```python
from build123d import *

# Parameters (mm, degrees)
F0_W     = 129.536152
F0_H     = 24.80902
F2_DEPTH = 2
F1_W     = 2.46322
F1_H     = 3.985553
F1_W_2   = 9.229143
F1_H_2   = 15.286758
F1_W_3   = 2.812087
F1_H_3   = 9.482866
F1_W_4   = 2.463219
F1_H_4   = 5.571315
F3_DEPTH = 1.5


with BuildPart() as f2:
    # F0 (on Top) → F2 (new body)
    with BuildSketch(Plane.XY):
        Rectangle(F0_W, F0_H)
    extrude(amount=-F2_DEPTH)

    # F1 (on Top) → F3 (join)
    with BuildSketch(Plane.XY):
        Polygon((-53.720365, 7.334459), (-53.720365, -1.440098), (-56.82846, 7.334459), (-59.999987, 7.334459), (-59.999987, -7.952299), (-56.997608, -7.952299), (-56.997608, 0.822258), (-53.868369, -7.952299), (-50.696842, -7.952299), (-50.696842, 7.334459), align=None)
        Polygon((-43.87806, -7.952299), (-43.87806, -5.055639), (-44.935236, -5.055639), (-44.935236, 4.437799), (-43.87806, 4.437799), (-43.87806, 7.334459), (-49.195653, 7.334459), (-49.195653, 4.437799), (-48.138477, 4.437799), (-48.138477, -5.055639), (-49.195653, -5.055639), (-49.195653, -7.952299), align=None)
        Polygon((-36.541261, -2.698137), (-36.541261, -5.055639), (-39.289917, -5.055639), (-39.289917, 4.427227), (-33.898322, 4.427227), (-33.898322, 7.334459), (-42.503731, 7.334459), (-42.503731, -7.952299), (-33.369735, -7.952299), (-33.369735, 0.018804), (-37.841588, 0.018804), (-37.841588, -2.698137), align=None)
        Polygon((-24.478888, 7.334459), (-31.90026, 7.334459), (-31.90026, -7.952299), (-24.37317, -7.952299), (-24.37317, -5.055639), (-28.686446, -5.055639), (-28.686446, -1.376668), (-24.690323, -1.376668), (-24.690323, 1.477707), (-28.728733, 1.477707), (-28.728733, 4.427227), (-24.478888, 4.427227), align=None)
        Polygon((-23.199705, 7.334459), (-23.199705, -7.952299), (-15.514039, -7.952299), (-15.514039, -5.055639), (-19.996463, -5.055639), (-19.996463, 7.334459), align=None)
        Polygon((-3.409379, -3.19501), (-3.409379, -5.055639), (-5.988887, -5.055639), (-5.988887, 4.427227), (-3.409379, 4.427227), (-3.409379, 1.562281), (-0.195565, 1.562281), (-0.195565, 7.334459), (-6.919202, 7.334459), (-9.202701, 5.23068), (-9.202701, -7.952299), (-2.309916, -7.952299), (-0.195565, -5.837948), (-0.195565, -3.19501), align=None)
        Polygon((5.1326, -2.423271), (7.035516, -7.952299), (10.24933, -7.952299), (8.219553, -2.380984), (9.953321, -2.380984), (9.953321, 7.334459), (3.409404, 7.334459), (1.083618, 5.177821), (1.083618, -7.952299), (4.286859, -7.952299), (4.286859, -2.423271), align=None)
        with Locations((5.518469, 2.43445)):
            Rectangle(F1_W, F1_H, mode=Mode.SUBTRACT)
        with Locations((16.047938, -0.30892)):
            Rectangle(F1_W_2, F1_H_2)
        with Locations((16.053224, -0.314206)):
            Rectangle(F1_W_3, F1_H_3, mode=Mode.SUBTRACT)
        Polygon((22.068553, -7.952299), (25.271795, -7.952299), (25.271795, -4.072465), (30.938256, -4.072465), (30.938256, 7.334459), (24.383768, 7.334459), (22.068553, 5.177821), align=None)
        with Locations((26.503404, 1.641569)):
            Rectangle(F1_W_4, F1_H_4, mode=Mode.SUBTRACT)
        Polygon((32.302012, 7.334459), (32.302012, -7.952299), (39.987679, -7.952299), (39.987679, -5.055639), (35.505254, -5.055639), (35.505254, 7.334459), align=None)
        Polygon((48.78338, 7.334459), (41.362008, 7.334459), (41.362008, -7.952299), (48.889098, -7.952299), (48.889098, -5.055639), (44.575821, -5.055639), (44.575821, -1.376668), (48.571945, -1.376668), (48.571945, 1.477707), (44.533534, 1.477707), (44.533534, 4.427227), (48.78338, 4.427227), align=None)
        Polygon((60.000013, 7.334459), (56.66991, 7.334459), (55.063003, 2.598313), (53.582958, 7.334459), (50.273998, 7.334459), (53.477239, -2.106119), (53.477239, -7.952299), (57.278849, -7.952299), (57.278849, -2.106119), align=None)
    extrude(amount=F3_DEPTH)


solid = f2.part
```
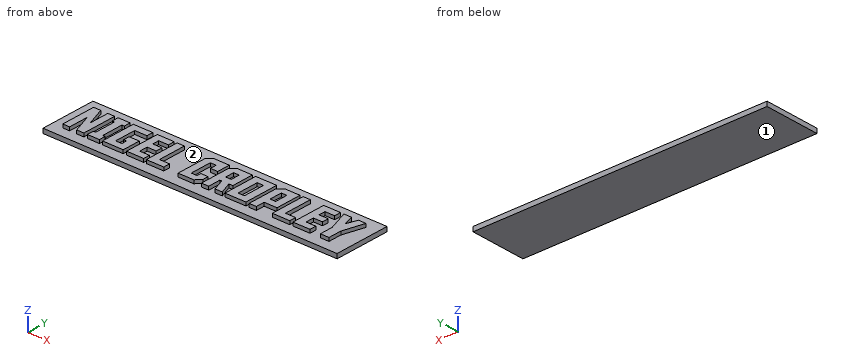
Part model, mm, in its own coordinate system. Face numbers are marked on the shaded views. Round coordinates to 2 decimals unless told otherwise and drop trailing zeros. Loops run counter-clockwise (first coordinate to the right, second up) from the corner with the lowest first, then second, coordinate; pieces in that order, holes last. Notation, with made-up numbers: (45, -24) -> (77, -24) arc R23 ccw to (77, -15) -> close; hole circle Ø8 at (-8, -25.75). An arc over 180 degrees is marked (long way). Use one line per item in the form item = value. Start each with the question number.
Item 1: Band-saw the part on C-C (x = 38). List the corners of the cut face in (y, z), plus the area to 3 significant figures.
Item 2: Band-saw the part on B-B (x = 16). List the corners of the cut face in (y, z), plus the area to 3 significant figures.
Item 3: Band-saw the part on A-A (z = 0.7). Give the number of separate pieces and of enclosed holes in the cut face, plus the area to 3 significant figures.
Item 4: Drill centre lines: line 1 along Z through (x, y) = (-11.5, 2.5); line 2 along Y through (x, z) = (39.5, 0.7); line 3 along Y through (x, z) = (-51, 1.25). Where is each one in solid material? Low to high.
Item 5: Two-plate mould, pull along X, no slides. Class the marked faces 1 and 2: released by +X, released by -X, zero draft, split by the parting line, or undercut.
Item 6: Drop flat-ended pins along their axis: pin 1 Ø1.4 at (x, z) = (-37.5, 1) entering from -Y; pin 2 Ø1.6 at (y, z) = (6.5, 1) entering from -X; pin 3 Ø1.2 at (y, z) = (-7, 1) entering from +X. Give the stop position or say it passes through.
Data:
q1.outline = (-12.4, -2) -> (12.4, -2) -> (12.4, 0) -> (-5.06, 0) -> (-5.06, 1.5) -> (-7.95, 1.5) -> (-7.95, 0) -> (-12.4, 0) -> close
q1.area = 54.0 mm^2
q2.outline = (-12.4, -2) -> (12.4, -2) -> (12.4, 0) -> (7.33, 0) -> (7.33, 1.5) -> (4.43, 1.5) -> (4.43, 0) -> (-5.06, 0) -> (-5.06, 1.5) -> (-7.95, 1.5) -> (-7.95, 0) -> (-12.4, 0) -> close
q2.area = 58.3 mm^2
q3.separate_pieces = 12
q3.enclosed_holes = 3
q3.area = 1,070 mm^2
q4.line_1 = -2 to 0
q4.line_2 = -7.95 to -5.06
q4.line_3 = -7.95 to 7.33
q5.face_1 = zero draft
q5.face_2 = undercut
q6.pin_1 = -7.95
q6.pin_2 = -60
q6.pin_3 = 57.28
